Autodesk Inventor part; units mm, degrees
ref_plane "YZ Plane" through (0, 0, 0) normal (1, 0, 0) x (0, 1, 0)
ref_plane "XZ Plane" through (0, 0, 0) normal (0, 1, 0) x (-1, 0, 0)
ref_plane "XY Plane" through (0, 0, 0) normal (0, 0, 1) x (1, 0, 0)
sketch "Sketch1" plane through (0, 0, 0) normal (0, 1, 0) x (-1, 0, 0)
  line L0 (4.6826, 5.0563) -> (-4.3174, 5.0563)
  line L1 (-4.3174, 5.0563) -> (-4.3174, -5.9437)
  line L2 (-4.3174, -5.9437) -> (-0.3174, -5.9437)
  line L3 (4.6826, 5.0563) -> (-0.3174, -5.9437)
  point P0 (0, 0)
  dimension "d0" = 11
  dimension "d1" = 9
  dimension "d2" = 4
extrude "Extrusion1" add sketch "Sketch1" along normal blind 10
sketch "Sketch2" plane through (4.3174, 0, 5.0563) normal (1, 0, 0) x (0, 0, -1)
  line L0 (5.5037, 7.3678) -> (7.55, 3.815)
  line L1 (7.55, 3.815) -> (5.4963, 2.6322)
  line L2 (5.4963, 2.6322) -> (3.45, 6.185)
  line L3 (3.45, 6.185) -> (5.5037, 7.3678)
  line L4 (3.45, 6.185) -> (7.55, 6.185)
  line L5 (7.55, 6.185) -> (7.55, 3.815)
  line L6 (7.55, 3.815) -> (3.45, 3.815)
  line L7 (3.45, 3.815) -> (3.45, 6.185)
  line L8 (5.5037, 7.3678) -> (7.55, 6.185)
  line L9 (3.45, 3.815) -> (5.4963, 2.6322)
  line L10 (0, 0) -> (11, 0)
  line L11 (11, 0) -> (11, 10)
  line L12 (0, 10) -> (11, 10)
  line L13 (0, 0) -> (0, 10)
  line L14 (3.45, 6.185) -> (7.55, 3.815)
  line L15 (3.45, 3.815) -> (7.55, 6.185)
  line L16 (5.5037, 7.3678) -> (5.4963, 2.6322)
  point P0 (5.0563, 0)
  point P1 (11, 0)
  point P2 (5.5, 5)
  dimension "d6" = 4.1
  dimension "d7" = 2.37
  dimension "d8" = 4.1
  dimension "d9" = 2.37
  dimension "d11" = 5
  dimension "d12" = 5.5
extrude "Extrusion2" cut sketch "Sketch2" against normal through all contours L8 L4 L0 | L16 L4 L3 | L0 L4 L16 | L4 L15 L0 | L0 L15 L16 L4 | L14 L15 L2 | L2 L15 L7 | L4 L16 L14 | L5 L0 L15 | L0 L14 L15 | L15 L16 L6 L2 | L2 L6 L15 | L6 L2 L9 | L14 L6 L16 | L1 L16 L6 | L6 L16 L2
sketch "Sketch3" plane through (0, 10, 0) normal (0, 1, 0) x (1, 0, 0)
  line L0 (-4.6826, -5.0563) -> (4.3174, -5.0563)
  line L1 (4.3174, -5.0563) -> (4.3174, 5.9437)
  line L2 (4.3174, 5.9437) -> (0.3174, 5.9437)
  line L3 (0.3174, 5.9437) -> (-4.6826, -5.0563)
  line L4 (0.3399, 17.9475) -> (4.3174, 17.9475)
  line L5 (4.3174, 17.9475) -> (4.3174, -17.0525)
  line L6 (4.3174, -17.0525) -> (0.3399, -17.0525)
  line L7 (0.3399, -17.0525) -> (0.3399, 17.9475)
  line L8 (4.3174, -1.6063) -> (-3.1144, -1.6063)
  line L9 (4.3174, 2.4937) -> (-1.2508, 2.4937)
  line L10 (4.3174, 0.4475) -> (-2.1809, 0.4475)
  line L11 (4.3174, 17.9475) -> (14.3174, 17.9475)
  line L12 (14.3174, 17.9475) -> (14.3174, -17.0525)
  line L13 (14.3174, -17.0525) -> (4.3174, -17.0525)
  line L14 (4.3174, -17.0525) -> (4.3174, 17.9475)
  line L15 (4.3174, 6.4475) -> (10.3174, 6.4475)
  line L16 (10.3174, 6.4475) -> (10.3174, -5.5525)
  line L17 (10.3174, -5.5525) -> (4.3174, -5.5525)
  line L18 (4.3174, -5.5525) -> (4.3174, 6.4475)
  point P0 (0, 0)
  dimension "d15" = 35
  dimension "d16" = 17.5
  dimension "d17" = 10
  dimension "d18" = 6
  dimension "d19" = 6
  dimension "d20" = 12
extrude "Extrusion3" add sketch "Sketch3" along normal blind 1 contours L3 L8 L7 L0 | L7 L8 L1 L0 | L0 L5 L6 L7 | L3 L10 L7 L8 | L7 L10 L1 L8 | L3 L9 L7 L10 | L17 L16 L15 L5 L11 L12 L13 | L7 L9 L1 L10 | L3 L2 L7 L9 | L7 L2 L1 L9 | L7 L4 L5 L2
sketch "Sketch4" plane through (0, 10, 0) normal (0, -1, 0) x (1, 0, 0)
  line L0 (4.3174, -5.9437) -> (0.3399, -5.9437)
  line L1 (0.3399, -17.9475) -> (0.3399, -5.9437)
  line L2 (14.3174, -17.9475) -> (0.3399, -17.9475)
  line L3 (14.3174, 17.0525) -> (14.3174, -17.9475)
  line L4 (0.3399, 17.0525) -> (14.3174, 17.0525)
  line L5 (0.3399, 5.0563) -> (0.3399, 17.0525)
  line L6 (0.3399, 5.0563) -> (4.3174, 5.0563)
  line L7 (4.3174, 5.0563) -> (4.3174, 5.5525)
  line L8 (4.3174, 5.5525) -> (10.3174, 5.5525)
  line L9 (10.3174, 5.5525) -> (10.3174, -6.4475)
  line L10 (10.3174, -6.4475) -> (4.3174, -6.4475)
  line L11 (4.3174, -6.4475) -> (4.3174, -5.9437)
  line L12 (0.3399, 17.0525) -> (14.3174, 17.0525)
  line L13 (14.3174, -17.9475) -> (10.3174, -17.9475)
  line L14 (10.3174, -17.9475) -> (10.3174, 17.0525)
  line L15 (10.3174, 17.0525) -> (14.3174, 17.0525)
  line L16 (14.3174, 17.0525) -> (14.3174, -17.9475)
  point P0 (0, 0)
  dimension "d23" = 4
extrude "Extrusion4" add sketch "Sketch4" along normal blind 10 contours L9 L14 L4 L3 L2
sketch "Sketch5" plane through (14.3174, 11, 17.0525) normal (1, 0, 0) x (0, 0, -1)
  line L0 (5.2643, -5.4963) -> (8.8172, -3.45)
  line L1 (8.8172, -3.45) -> (10, -5.5037)
  line L2 (10, -5.5037) -> (6.4472, -7.55)
  line L3 (6.4472, -7.55) -> (5.2643, -5.4963)
  line L4 (6.4472, -7.55) -> (6.4472, -3.45)
  line L5 (6.4472, -3.45) -> (8.8172, -3.45)
  line L6 (8.8172, -3.45) -> (8.8172, -7.55)
  line L7 (8.8172, -7.55) -> (6.4472, -7.55)
  line L8 (5.2643, -5.4963) -> (6.4472, -3.45)
  line L9 (8.8172, -7.55) -> (10, -5.5037)
  line L10 (19.2733, 12.7) -> (12, 12.7)
  line L11 (25, -5.5037) -> (28.5528, -3.4574)
  line L12 (28.5528, -3.4574) -> (29.7357, -5.5112)
  line L13 (29.7357, -5.5112) -> (26.1828, -7.5574)
  line L14 (26.1828, -7.5574) -> (25, -5.5037)
  line L15 (26.1828, -7.5574) -> (26.1828, -3.4574)
  line L16 (26.1828, -3.4574) -> (28.5528, -3.4574)
  line L17 (28.5528, -3.4574) -> (28.5528, -7.5574)
  line L18 (28.5528, -7.5574) -> (26.1828, -7.5574)
  line L19 (25, -5.5037) -> (26.1828, -3.4574)
  line L20 (28.5528, -7.5574) -> (29.7357, -5.5112)
  line L21 (0, 0) -> (35, 0)
  line L22 (0, 0) -> (0, -11)
  line L23 (35, -11) -> (35, 0)
  line L24 (6.4472, -7.55) -> (8.8172, -3.45)
  line L25 (6.4472, -3.45) -> (8.8172, -7.55)
  line L26 (10, -5.5037) -> (5.2643, -5.4963)
  line L27 (26.1828, -3.4574) -> (28.5528, -7.5574)
  line L28 (26.1828, -7.5574) -> (28.5528, -3.4574)
  line L29 (25, -5.5037) -> (29.7357, -5.5112)
  line L30 (35, -11) -> (35, 0)
  line L31 (0, 0) -> (35, 0)
  line L32 (0, 0) -> (0, -11)
  line L33 (35, -11) -> (0, -11)
  line L34 (19.5463, -7.185) -> (17.4926, -8.3678)
  line L35 (17.4926, -8.3678) -> (15.4463, -7.185)
  line L36 (15.4463, -7.185) -> (15.4463, -4.815)
  line L37 (15.4463, -4.815) -> (17.5, -3.6322)
  line L38 (17.5, -3.6322) -> (19.5463, -4.815)
  line L39 (19.5463, -4.815) -> (19.5463, -7.185)
  line L40 (15.4463, -7.185) -> (19.5463, -4.815)
  line L41 (15.4463, -4.815) -> (19.5463, -7.185)
  line L42 (19.5463, -7.185) -> (17.4926, -8.3678)
  line L43 (17.5, -3.6322) -> (17.4926, -8.3678)
  circle A0 centre (17.4963, -6) radius 1.5
  point P0 (17.0525, -11)
  point P1 (11, 0)
  point P2 (7.6322, -5.5)
  point P3 (27.3678, -5.5074)
  dimension "d26" = 4.1
  dimension "d27" = 2.37
  dimension "d28" = 4.1
  dimension "d29" = 2.37
  dimension "d31" = 4.1
  dimension "d32" = 2.37
  dimension "d33" = 4.1
  dimension "d34" = 2.37
  dimension "d36" = 10
  dimension "d37" = 10
  dimension "d38" = 5.5
  dimension "d39" = 3
extrude "Extrusion5" cut sketch "Sketch5" against normal up to surface (4 mm away) contours L8 L4 L0 | L26 L4 L3 | L0 L4 L26 | L4 L25 L0 | L0 L25 L26 L4 | L24 L25 L2 | L2 L25 L7 | L4 L26 L24 | L5 L0 L25 | L0 L24 L25 | L25 L26 L6 L2 | L2 L6 L25 | L6 L2 L9 | L24 L6 L26 | L1 L26 L6 | L6 L26 L2 | L19 L15 L11 | L29 L15 L14 | L11 L15 L29 | L15 L27 L11 | L11 L27 L29 L15 | L28 L27 L13 | L13 L27 L18 | L15 L29 L28 | L16 L11 L27 | L11 L28 L27 | L27 L29 L17 L13 | L13 L17 L27 | L17 L13 L20 | L28 L17 L29 | L12 L29 L17 | L17 L29 L13 | A0 L43 L41 | L41 L40 A0 | A0 L40 L43 | L40 L43 A0 | L40 A0 L41 | L41 A0 L43
sketch "Sketch6" plane through (14.3174, 11, 17.0525) normal (1, 0, 0) x (0, 0, -1)
  circle A0 centre (17.4963, -6) radius 1.5
  circle A1 centre (17.4963, -6) radius 3
  point P0 (17.0525, -11)
  dimension "d42" = 6
extrude "Extrusion6" cut sketch "Sketch6" against normal blind 2
sketch "Sketch7" plane through (0, 11, 0) normal (0, 1, 0) x (1, 0, 0)
  line L0 (4.3174, 6.4475) -> (4.3174, -5.5525)
  line L1 (4.3174, 6.4475) -> (10.3174, 6.4475)
  line L2 (10.3174, 6.4475) -> (10.3174, -5.5525)
  line L3 (10.3174, -5.5525) -> (4.3174, -5.5525)
  line L4 (0.3399, 5.9437) -> (0.3174, 5.9437)
  line L5 (0.3174, 5.9437) -> (-4.6826, -5.0563)
  line L6 (-4.6826, -5.0563) -> (0.3399, -5.0563)
  line L7 (0.3399, -5.0563) -> (0.3399, -17.0525)
  line L8 (0.3399, -17.0525) -> (14.3174, -17.0525)
  line L9 (14.3174, -17.0525) -> (14.3174, 17.9475)
  line L10 (14.3174, 17.9475) -> (0.3399, 17.9475)
  line L11 (0.3399, 17.9475) -> (0.3399, 5.9437)
  point P0 (0, 0)
extrude "Extrusion7" add sketch "Sketch7" along normal blind 3
ref_plane "Work Plane1" through (-4.6826, 7, 5.0563) normal (-1, 0, 0) x (0, 0, 1)
sketch "Sketch8" plane through (-4.6826, 7, 5.0563) normal (-1, 0, 0) x (0, 0, 1)
  circle A0 centre (-5.5, -2) radius 3
  circle A1 centre (-5.5, -2) radius 4.211
  point P0 (-5.0563, -7)
extrude "Extrusion8" cut sketch "Sketch8" against normal blind 3 contours A0 | A1
sketch "Sketch9" plane through (0.3399, 10, 5.0563) normal (-1, 0, 0) x (0, 0, 1)
  line L0 (0, 0) -> (0, 4)
  line L1 (0, 0) -> (11.9963, 0)
  line L2 (11.9963, 0) -> (11.9963, 4)
  line L3 (0, 4) -> (11.9963, 4)
  point P0 (-5.0563, -10)
extrude "Extrusion9" add sketch "Sketch9" along normal up to surface (5.0225 mm away)
equation "\"d16\" = 0.5 * d15"
properties part number "world_cam_mount"
The model under review builds one solid part; all positions refer to its coordinate system, in mm. A direction names the side the tool comes from. Give positions to 0.01 mm unless a question says otherwise; leave off trailing zeros. Loops run counter-clockwise (first coordinate to the right, second up) from the corner with the lowest first, then second, coordinate; pieces in that order, holes last. Notation, with made-up numbers: (-4, 36.25) -> (49, 36.25) arc R15 cw to (49, 48.25) -> close; hole circle Ø8 at (33, 6). An arc over 180 degrees is marked (long way). Answer as a JSON object with one key per item and string values. Group by question number.
Q1. Take a section at A-A (x = 5.25). Write out the cut boundary in (y, z).
Q2. Take a section at C-C (y = 5). State how many separate pieces and enclosed holes the cut face has, plus the area to 3 significant figures.
Q3. Take a section at B-B (z = -11). Write out the cut boundary in (x, y), plus the area to 3 significant figures.
Q4. Take a section at D-D (y = 1.5). Write out the cut boundary in (x, z), plus the area to 3 significant figures.
Q5. Tool access review of faces 1 (the flat face through (12.345, 4.462, 11.188)), 2 (the flat face through (1.359, 6.785, -1.456)), 3 (the cylindrical face through (13.331, 2.071, 0.207)), 4 (the flat face through (4.317, 7, -2)), 5 (the flat face through (3, 10, 11)): name each direction out of +Z, -Z, +X, -X, +Y, -Y from which nothing blocks a thin tool from reaching the whole face with its end or side.
Q6. Insertion check: pin 1 (0.7 mm diameter, centred on x = 12, z = -10, fed in from -Y); pin 2 (5 mm diameter, centred on y = 6, z = -13.5, fed in from -X); pin 3 (1.2 mm diameter, centred on x = 1, y = 4.5, fed in from -Z); pin 4 (6 mm diameter, centred on x = 4.5, z = 11, fed in from -Y). Each pin has a flat end and moves straight along its axis. Give the tip position at first contact, or say it passes through.
Q7. Draft analysis for pull direction X (two halves, no side actions). For faces 6 (the flat face through (12.345, 6.513, 11.205)), 7 (the flat face through (10.317, 7, -1)), 8 (the flat face through (-1.683, 5, 2)), state which applies: pulls with the +X half, pulls with the -X half, needs draft (parallel to the pull), parting line crosses it, or undercut.
Q8. Wall thickness on line 1 along Z through (x, y) = (7.5, 10.75); line 2 along Z through (x, y) = (-1.25, 10.5); line 3 along X through (y, z) = (13, -13): over which ranges is each line inside the solid? List them lowest first.
Answer below:
{
 "1": {"outline": "(10, -17.95) -> (14, -17.95) -> (14, -6.45) -> (10, -6.45) -> close; (10, 5.55) -> (14, 5.55) -> (14, 17.05) -> (10, 17.05) -> close"},
 "2": {"separate pieces": "6", "enclosed holes": "0", "area": "129 mm2"},
 "3": {"outline": "(0.34, 10) -> (10.32, 10) -> (10.32, 7.54) -> (14.32, 7.54) -> (14.32, 14) -> (0.34, 14) -> close; (10.32, 0) -> (14.32, 0) -> (14.32, 3.44) -> (10.32, 3.44) -> close", "area": "79.5 mm2"},
 "4": {"outline": "(-4.68, 5.06) -> (-3.25, 1.9) -> (-1.68, 1.9) -> (-1.68, -1.54) -> (0.32, -5.94) -> (4.32, -5.94) -> (4.32, 5.06) -> close; (10.32, -17.95) -> (14.32, -17.95) -> (14.32, 17.05) -> (10.32, 17.05) -> close", "area": "209 mm2"},
 "5": {"face 1": "+X, -X", "face 2": "-X", "face 3": "+X", "face 4": "+Y, -Y", "face 5": "+Z, -X, -Y"},
 "6": {"pin 1": "stops at y = 0", "pin 2": "stops at x = 10.32", "pin 3": "stops at z = -5.94", "pin 4": "stops at y = 10"},
 "7": {"face 6": "needs draft", "face 7": "undercut", "face 8": "pulls with the -X half"},
 "8": {"line 1": "z = -17.95 to -6.45, 5.55 to 17.05", "line 2": "z = -2.5 to 17.05", "line 3": "x = 0.34 to 14.32"}
}
